Read the model definition and answer for the solid it produces. Units are mm, in the model's axes. A direction names the side the tool comes from. Coordinates: 2 decimals unless noted, no trailing zeros. Order: outer loops, then holes, each group sorted by start corner. A loop starts at its lowest first (then second) coordinate and runs counter-clockwise, first axis right, second up.
from build123d import *

# Parameters (mm, degrees)
SKETCH2_W            = 15.8
SKETCH2_H            = 15.8
BOSS_EXTRUDE2_DEPTH  = 4.2
SKETCH4_W            = 13.4
SKETCH4_H            = 13.4
CUT_EXTRUDE1_DEPTH   = 3
SKETCH6_R            = 2.41
BOSS_EXTRUDE4_DEPTH  = 1.8
LPATTERN1_COUNT      = 2
LPATTERN1_PITCH      = 8
LPATTERN1_COUNT_DIR2 = 2
LPATTERN1_PITCH_DIR2 = 8
SKETCH8_R            = 5.25
CUT_EXTRUDE2_DEPTH   = 0.1
BOSS_EXTRUDE9_DEPTH  = 3
CUT_EXTRUDE3_DEPTH   = 3
SKETCH20_W           = 3
SKETCH20_H           = 1.35
CUT_EXTRUDE4_DEPTH   = 1.25
CIRPATTERN3_COUNT    = 4


with BuildPart() as part:
    # Sketch2 → Boss-Extrude2 (new body)
    with BuildSketch(Plane(origin=(0, 0, 0), x_dir=(1, 0, 0), z_dir=(0, 1, 0))):
        with Locations((7.9, 7.9)):
            Rectangle(SKETCH2_W, SKETCH2_H)
    extrude(amount=-BOSS_EXTRUDE2_DEPTH)

    # Sketch4 → Cut-Extrude1 (cut)
    with BuildSketch(Plane(origin=(0, 0, 0), x_dir=(1, 0, 0), z_dir=(0, 1, 0))):
        with Locations((7.9, 7.9)):
            Rectangle(SKETCH4_W, SKETCH4_H)
    extrude(amount=-CUT_EXTRUDE1_DEPTH, mode=Mode.SUBTRACT)

    # Sketch6 → Boss-Extrude4 (add)
    with BuildSketch(Plane(origin=(0, -4.2, 0), x_dir=(-1, 0, 0), z_dir=(0, -1, 0))):
        with Locations((-11.9, 11.9)):
            Circle(SKETCH6_R)
    boss_extrude4 = extrude(amount=BOSS_EXTRUDE4_DEPTH)

    # LPattern1: Boss-Extrude4 2 × 2
    with Locations(*[(-j * LPATTERN1_PITCH_DIR2, 0, i * LPATTERN1_PITCH) for i in range(LPATTERN1_COUNT) for j in range(LPATTERN1_COUNT_DIR2) if (i, j) != (0, 0)]):
        add(boss_extrude4)

    # Sketch8 → Cut-Extrude2 (cut)
    with BuildSketch(Plane(origin=(0, -3, 0), x_dir=(1, 0, 0), z_dir=(0, 1, 0))):
        with Locations((7.9, 7.9)):
            Circle(SKETCH8_R)
    extrude(amount=-CUT_EXTRUDE2_DEPTH, mode=Mode.SUBTRACT)

    # Sketch11 → Boss-Extrude9 (add)
    with BuildSketch(Plane(origin=(0, -3, 0), x_dir=(1, 0, 0), z_dir=(0, 1, 0))):
        with BuildLine():
            Line((7.899999971, 14.6), (1.2, 14.6))
            Line((1.2, 14.6), (1.2, 7.9))
            ThreePointArc((1.2, 7.9), (3.162384556, 12.637615424), (7.899999971, 14.6))
        make_face()
        with BuildLine():
            Line((14.6, 14.6), (7.899999971, 14.6))
            ThreePointArc((7.899999971, 14.6), (12.637615424, 12.637615444), (14.6, 7.9))
            Line((14.6, 7.9), (14.6, 14.6))
        make_face()
        with BuildLine():
            ThreePointArc((7.900000011, 1.2), (3.16238457, 3.162384562), (1.2, 7.9))
            Line((1.2, 7.9), (1.2, 1.2))
            Line((1.2, 1.2), (7.900000011, 1.2))
        make_face()
        with BuildLine():
            Line((14.6, 1.2), (14.6, 7.9))
            ThreePointArc((14.6, 7.9), (12.637615438, 3.16238457), (7.900000011, 1.2))
            Line((7.900000011, 1.2), (14.6, 1.2))
        make_face()
    extrude(amount=BOSS_EXTRUDE9_DEPTH)

    # Sketch12 → Cut-Extrude3 (cut)
    with BuildSketch(Plane(origin=(0, 0, 0), x_dir=(1, 0, 0), z_dir=(0, 1, 0))):
        Polygon((3.162384566, 12.637615434), (2.455277785, 13.344722215), (1.394617613, 12.284062043), (2.101724394, 11.576955262), align=None)
        with BuildLine():
            ThreePointArc((2.221981276, 11.45669838), (2.658816927, 12.073727351), (3.162384566, 12.637615434))
            Line((3.162384566, 12.637615434), (2.101724394, 11.576955262))
            Line((2.101724394, 11.576955262), (2.221981276, 11.45669838))
        make_face()
        with BuildLine():
            Line((4.223044738, 13.698275606), (3.162384566, 12.637615434))
            ThreePointArc((3.162384566, 12.637615434), (3.726272649, 13.141183073), (4.34330162, 13.578018724))
            Line((4.34330162, 13.578018724), (4.223044738, 13.698275606))
        make_face()
        Polygon((3.515937957, 14.405382387), (2.455277785, 13.344722215), (3.162384566, 12.637615434), (4.223044738, 13.698275606), align=None)
        with BuildLine():
            ThreePointArc((4.34330162, 13.578018724), (3.726272649, 13.141183073), (3.162384566, 12.637615434))
            ThreePointArc((3.162384566, 12.637615434), (2.658816927, 12.073727351), (2.221981276, 11.45669838))
            Line((2.221981276, 11.45669838), (2.423581348, 11.255098309))
            Line((2.423581348, 11.255098309), (4.544901691, 13.376418652))
            Line((4.544901691, 13.376418652), (4.34330162, 13.578018724))
        make_face()
        with BuildLine():
            ThreePointArc((14.6, 7.9), (11.145005458, 13.761735202), (4.34330162, 13.578018724))
            Line((4.34330162, 13.578018724), (4.544901691, 13.376418652))
            Line((4.544901691, 13.376418652), (2.423581348, 11.255098309))
            Line((2.423581348, 11.255098309), (2.221981276, 11.45669838))
            ThreePointArc((2.221981276, 11.45669838), (6.049692654, 1.460561925), (14.6, 7.9))
        make_face()
    cut_extrude3 = extrude(amount=-CUT_EXTRUDE3_DEPTH, mode=Mode.SUBTRACT)

    # Sketch20 → Cut-Extrude4 (cut)
    with BuildSketch(Plane(origin=(-5.444722215, 0, -5.444722215), x_dir=(0.707106781, 0, -0.707106781), z_dir=(0.707106781, 0, 0.707106781))):
        with Locations((11.172287143, -2.325)):
            Rectangle(SKETCH20_W, SKETCH20_H)
    cut_extrude4 = extrude(amount=-CUT_EXTRUDE4_DEPTH, mode=Mode.SUBTRACT)

    # CirPattern3: Cut-Extrude3, Cut-Extrude4 ×4 about axis
    cirpattern3_axis = Axis((7.9, 0, -7.9), (0, 1, 0))
    for i in range(1, CIRPATTERN3_COUNT):
        add(cut_extrude3.rotate(cirpattern3_axis, i * 360 / CIRPATTERN3_COUNT), mode=Mode.SUBTRACT)
        add(cut_extrude4.rotate(cirpattern3_axis, i * 360 / CIRPATTERN3_COUNT), mode=Mode.SUBTRACT)


solid = part.part
Q1. Each of these flat-tipped pins is pushed along its axis until it touches: P1, Ø1.5, axis at x = 14.5, z = -1.5, coming from the -Y side; P2, Ø7.5, axis at x = 4.5, z = -9, coming from the +Y side; P3, Ø2, axis at x = 4, z = -4, coming from the +Y side; P4, Ø3, axis at x = 8, z = -9, coming from the +Y side. Where does it stop, or does it pass through?
Q2. The part is cut by section D-D, the plane y = -2.4. Determine the outline of the cut face in (x, z).
Q3. The part is cut by section B-B, the plane x = 3.25. Determine the outline of the cut face in (y, z), then the cut area to 3 significant figures.
Q4. The part is cut by section A-A, the plane y = -0.95. Determine the outline of the cut face in (x, z), then the cut area to 3 significant figures.
Q5. Determine the mould class of faces 1 (the flat face through (1.545, -1.812, -12.134)), 2 (the flat face through (3.69, -1.81, -14.23)), 3 (the flat face through (8, -2, 0)), 4 (the flat face through (0, -2, -8)) for opening direction X: +X half, -X half, draft (parallel to the pull), parting line (faces both ways), or undercut.
Q6. Straight lines are drawn through the part: L1, parallel to Z at x = 1, y = -1.7; L2, parallel to X at y = -3.05, z = -7.9; L3, parallel to Z at x = 7.9, y = -3.05. For each, find the intervals that lie inside material, in ascending order.
Q7. Which of the six approach directions +Z, -Z, +X, -X, +Y, -Y give full straight-line access (tool end or side, diameter ignored) to faces 5 (the flat face through (1, 0, -8)), 6 (the flat face through (2.47, -0.81, -13.36)), 7 (the flat face through (12, -6, -12)), 8 (the cylindrical face through (1.6, -5.09, -4.62)), 9 (the flat face through (1.557, -2.316, -14.214))?
Q8. The part is cut by section C-C, the plane z = -7. Determine the outline of the cut face in (x, y), then the cut area to 3 significant figures.
Computed values:
1. P1: stops at y = -4.2
1. P2: stops at y = 0
1. P3: stops at y = -3
1. P4: stops at y = -3.1
2. outline: (0, -15.8) - (15.8, -15.8) - (15.8, 0) - (0, 0) - close; hole (0.51, -13.17) - (2.63, -15.29) - (4.34, -13.58) arc R6.7 ccw to (11.46, -13.58) - (13.17, -15.29) - (15.29, -13.17) - (13.58, -11.46) arc R6.7 ccw to (13.58, -4.34) - (15.29, -2.63) - (13.17, -0.51) - (11.46, -2.22) arc R6.7 ccw to (4.34, -2.22) - (2.63, -0.51) - (0.51, -2.63) - (2.22, -4.34) arc R6.7 ccw to (2.22, -11.46) - close
3. outline: (-6, -14.22) - (-4.2, -14.22) - (-4.2, -15.8) - (0, -15.8) - (0, -14.14) - (-1.65, -14.14) - (-1.65, -14.67) - (-3, -14.67) - (-3, -10.34) - (-3.1, -10.34) - (-3.1, -5.46) - (-3, -5.46) - (-3, -1.13) - (-1.65, -1.13) - (-1.65, -1.66) - (0, -1.66) - (0, 0) - (-4.2, 0) - (-4.2, -1.58) - (-6, -1.58) - (-6, -6.22) - (-4.2, -6.22) - (-4.2, -9.58) - (-6, -9.58) - close
3. area: 43.7 mm2
4. outline: (0, -15.8) - (15.8, -15.8) - (15.8, 0) - (0, 0) - close; hole (1.39, -12.28) - (3.52, -14.41) - (4.34, -13.58) arc R6.7 ccw to (11.46, -13.58) - (12.28, -14.41) - (14.41, -12.28) - (13.58, -11.46) arc R6.7 ccw to (13.58, -4.34) - (14.41, -3.52) - (12.28, -1.39) - (11.46, -2.22) arc R6.7 ccw to (4.34, -2.22) - (3.52, -1.39) - (1.39, -3.52) - (2.22, -4.34) arc R6.7 ccw to (2.22, -11.46) - close
4. area: 95.9 mm2
5. face 1: undercut
5. face 2: undercut
5. face 3: draft
5. face 4: -X half
6. L1: z = -15.8 to -13.66, -12.68 to -3.12, -2.14 to 0
6. L2: x = 0 to 2.65, 13.15 to 15.8
6. L3: z = -15.8 to -13.15, -2.65 to 0
7. face 5: +Z, -Z, +X, -X, +Y
7. face 6: +Y
7. face 7: +Z, -Z, +X, -X, -Y
7. face 8: -Y
7. face 9: none
8. outline: (0, -4.2) - (15.8, -4.2) - (15.8, 0) - (14.54, 0) - (14.54, -3) - (13.07, -3) - (13.07, -3.1) - (2.73, -3.1) - (2.73, -3) - (1.26, -3) - (1.26, 0) - (0, 0) - close
8. area: 25.5 mm2
